Here's how the part is built. I have some questions about the finished solid (model axes, mm). A direction names the side the tool comes from. Coordinates: 2 decimals unless noted, no trailing zeros. Loops run counter-clockwise (first coordinate to the right, second up) from the corner with the lowest first, then second, coordinate; pieces in that order, holes last. Notation, with made-up numbers: (-11, 16) -> (47, 16) arc R21 ccw to (47, 26) -> close; hole circle Ø4 at (20.5, 55). An arc over 180 degrees is marked (long way). Answer as a JSON object with one key per item and string values. Group by question number.
1) Which directions (+Z, -Z, +X, -X, +Y, -Y) give clear straight access to the entire face, cutting with the end or side of a thin tool? Please do faces 1 (the conical face through (-0.73, -1.404, -0.987)), 2 (the flat face through (1.2, -1.2, 1.27)).
2) I'm going to push flat-ended pins straight in: pin 1 (1 mm diameter, centred on y = -1.5, z = 9, fed in from -X); pin 2 (1 mm diameter, centred on y = 0, z = 4, fed in from -X); pin 3 (1.7 mm diameter, centred on x = 1, y = 1, fed in from -Z). Where does each tip first touch, or does it pass through?
3) I need wall thicknesses on probe 1 along Z at (x, y) = (1.55, 0.85); probe 2 along X at (y, z) = (-0.3, 0.25); probe 3 along Y at (x, z) = (0.6, 1). Which ranges of each line are inside material? Lowest first, please. Write a range as [from, to].
4) I want a section at A-A (z = 0.5). Write out the boundary of the cut face in (x, y).
```python
from build123d import *

# Parameters (mm, degrees)
SKETCH1_R           = 2.794
BOSS_EXTRUDE1_DEPTH = 1.27
BOSS_EXTRUDE1_TAPER = 1
SKETCH2_R           = 1.524
BOSS_EXTRUDE2_DEPTH = 9.23000005
BOSS_EXTRUDE2_TAPER = 1
SKETCH3_R           = 1.6
BOSS_EXTRUDE3_DEPTH = 2.1
BOSS_EXTRUDE3_TAPER = 1
FILLET1_R           = 0.2


with BuildPart() as part:
    # Sketch1 → Boss-Extrude1 (new body)
    with BuildSketch(Plane.XY):
        Circle(SKETCH1_R)
    extrude(amount=BOSS_EXTRUDE1_DEPTH, taper=BOSS_EXTRUDE1_TAPER)

    # Sketch2 → Boss-Extrude2 (add)
    with BuildSketch(Plane.XY.offset(1.27)):
        Circle(SKETCH2_R)
    extrude(amount=BOSS_EXTRUDE2_DEPTH, taper=BOSS_EXTRUDE2_TAPER)

    # Sketch3 → Boss-Extrude3 (add)
    with BuildSketch(Plane(origin=(0, 0, 0), x_dir=(-1, 0, 0), z_dir=(0, 0, -1))):
        Circle(SKETCH3_R)
    extrude(amount=BOSS_EXTRUDE3_DEPTH, taper=BOSS_EXTRUDE3_TAPER)

    # Sketch5 → Cut-Revolve4 (revolve, cut)
    with BuildSketch(Plane(origin=(0, 0, 0), x_dir=(1, 0, 0), z_dir=(0, 1, 0))):
        with BuildLine():
            Line((0, -10.50000005), (0, -9.94120005))
            ThreePointArc((0, -9.94120005), (0.736499476, -10.086324189), (1.36288975, -10.50000005))
            Line((1.36288975, -10.50000005), (1.36288975, -10.823922581))
            Line((1.36288975, -10.823922581), (0, -10.823922581))
            Line((0, -10.823922581), (0, -10.50000005))
        make_face()
    revolve(axis=Axis((0, 0, 1.27), (0, 0, 1)), mode=Mode.SUBTRACT)

    # Sketch6 → Revolve1 (revolve)
    with BuildSketch(Plane(origin=(0, 0, 0), x_dir=(1, 0, 0), z_dir=(0, 1, 0))):
        with BuildLine():
            Line((0, 2.3), (0, 2.1))
            Line((0, 2.1), (-1.563344364, 2.1))
            ThreePointArc((-1.563344364, 2.1), (-0.788042765, 2.249797078), (0, 2.3))
        make_face()
    revolve(axis=Axis((0, 0, -2.1), (0, 0, -1)))

    # Fillet1
    fillet1_edges = [part.edges().sort_by_distance(p)[0] for p in [
        (1.563344364, 0, -2.1),
    ]]
    fillet(fillet1_edges, radius=FILLET1_R)


solid = part.part
```
Determined:
{
 "1": {"face 1": "-Z", "face 2": "+Z"},
 "2": {"pin 1": "x = -0.96", "pin 2": "x = -1.49", "pin 3": "z = -2.27"},
 "3": {"probe 1": "[0, 1.27]", "probe 2": "[-2.77, 2.77]", "probe 3": "[-2.71, 2.71]"},
 "4": {"outline": "circle Ø5.57 at (0, 0)"}
}
